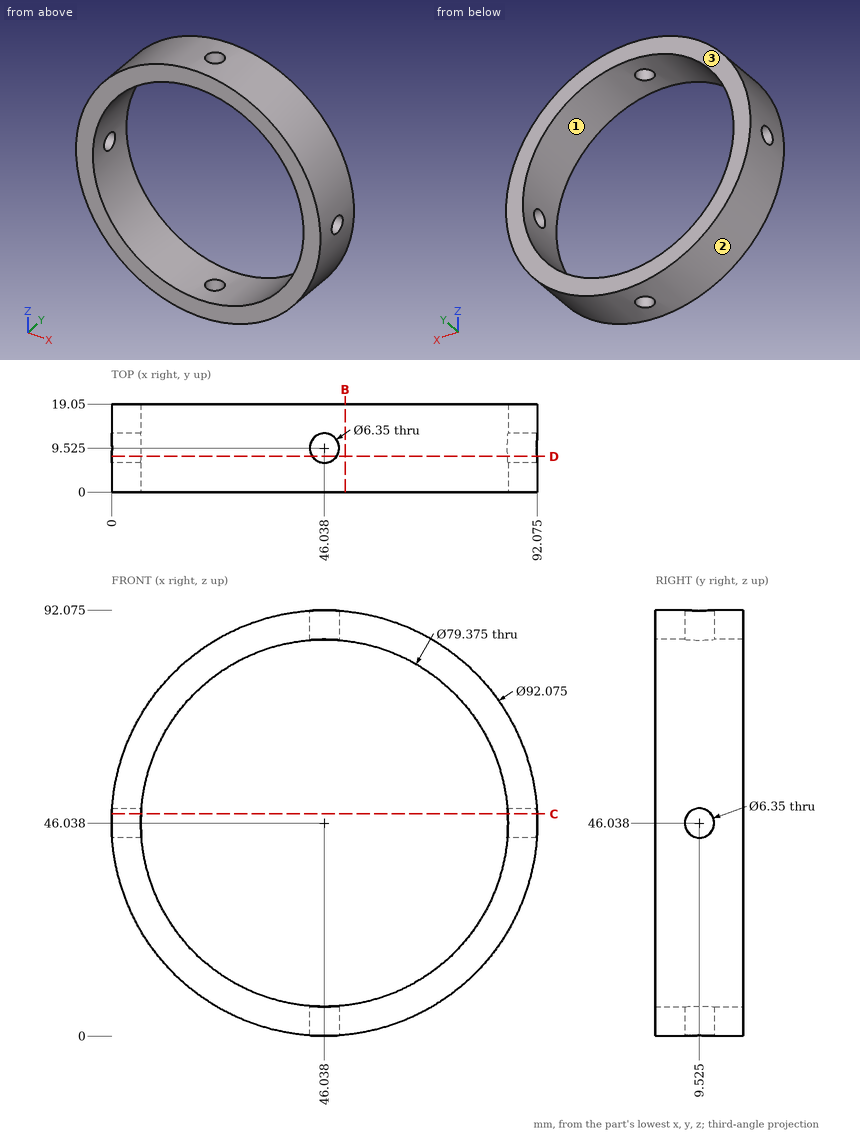
Input: dimensioned drawing with shaded views. Units: mm. Origin: part minimum x, y, z. Round coordinates to 2 decimals unless told otherwise and drop trailing zeros. Loops run counter-clockwise (first coordinate to the right, second up) from the corner with the lowest first, then second, coordinate; pieces in that order, holes last. Notation, with made-up numbers: M 89.5,25 L 136.5,25 A32 cw 136.5,52 Z; hole C 62,-13 d4. An arc over 180 degrees is marked long. One line per question, with ' | ' between items.
(1) Pull-direction query (Z, two-part tool) for the marked faces 1, 2 and 3; classes: +Z half, -Z half, draft (parallel to the pull), parting line (faces both ways), or undercut.
Check result:
face 1: undercut | face 2: parting line | face 3: draft
(2) Cut plane B-B on x = 50.5. Return the cut outline in (y, z), plus the area to 3 significant figures.
Check result:
outline: M 0,0.22 L 19.05,0.22 L 19.05,6.6 L 0,6.6 Z; M 0,85.47 L 19.05,85.47 L 19.05,91.86 L 0,91.86 Z | area: 243 mm2
(3) Material intervals for line 1 along Z through (x, y) = (70, 15.75) (1 decimal); line 2 along Z through (x, y) = (50, 1.75) (1 decimal); line 3 along X through (y, z) = (8.25, 36) (1 decimal), sorted ascending. Write a range as from..to.
Check result:
line 1: z = 6.7..14.4, 77.7..85.3 | line 2: z = 0.2..6.5, 85.5..91.9 | line 3: x = 1.1..7.6, 84.4..91
(4) Cut plane C-C on z = 48. Return the cut outline in (x, y).
Check result:
outline: M 0.04,0 L 6.4,0 L 6.4,7.03 L 0.04,7.03 Z; M 0.04,12.02 L 6.4,12.02 L 6.4,19.05 L 0.04,19.05 Z; M 85.68,0 L 92.03,0 L 92.03,7.03 L 85.68,7.03 Z; M 85.68,12.02 L 92.03,12.02 L 92.03,19.05 L 85.68,19.05 Z
(5) Cut plane D-D on y = 7.75. Return the cut outline in (x, z) (1 decimal).
Check result:
outline: M 0.1,43.4 A46 ccw 43.4,0.1 L 43.4,6.4 A39.7 cw 6.4,43.4 Z; M 0.1,48.7 L 6.4,48.7 A39.7 cw 43.4,85.6 L 43.4,92 A46 ccw Z; M 48.7,0.1 A46 ccw 92,43.4 L 85.6,43.4 A39.7 cw 48.7,6.4 Z; M 48.7,85.6 A39.7 cw 85.6,48.7 L 92,48.7 A46 ccw 48.7,92 Z
(6) Contact query for flat-ended pins moving along their axis: P1, Ø5, axis at x = 28, y = 13, coming from the -Z side; P2, Ø5, axis at x = 73.5, y = 16.5, coming from the +Z side; P3, Ø8, axis at x = 19, y = 13.5, coming from the +Z side (1 decimal); P4, Ø5.5, axis at x = 46.04, y = 9.53, coming from the +Z side. Output: stop coordinate, or through.
Check result:
P1: stops at z = 2.7 | P2: stops at z = 84.72 | P3: stops at z = 85.9 | P4: passes through
